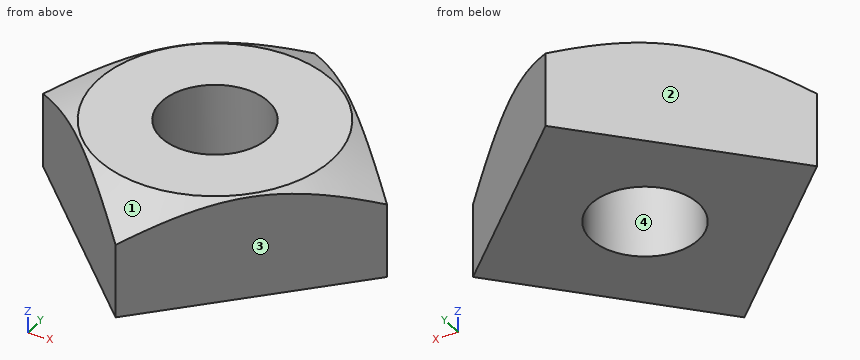
from build123d import *

# Parameters (mm, degrees)
SKETCH_7_R      = 1.229375
EXTRUDE_1_DEPTH = 2.4


with BuildPart() as part:
    # 草图7 → 凸台-拉伸1 (new body)
    with BuildSketch(Plane.XY):
        Polygon((-3.889087297, 0), (0, 3.889087297), (3.889087297, 0), (0, -3.889087297), align=None)
        Circle(SKETCH_7_R, mode=Mode.SUBTRACT)
    extrude(amount=-EXTRUDE_1_DEPTH)

    # 草图8 → 切除-旋转1 (revolve, cut)
    with BuildSketch(Plane(origin=(0, 0, 0), x_dir=(0, 0, -1), z_dir=(1, 0, 0))):
        Polygon((0.692820323, 3.889087297), (0, 2.689087297), (0, 3.889087297), align=None)
    revolve(axis=Axis((0, 0, 0), (0, 0, -1)), mode=Mode.SUBTRACT)


solid = part.part
For this review, take the finished solid that the model builds, in its own axes (mm). Face numbers are marked on the shaded views. Give positions to 0.01 mm unless a question says otherwise; leave off trailing zeros. Loops run counter-clockwise (first coordinate to the right, second up) from the corner with the lowest first, then second, coordinate; pieces in that order, holes last. Notation, with made-up numbers: (60.25, 55.25) -> (90.25, 55.25) arc R13 ccw to (90.25, 63.25) -> close; hole circle Ø7 at (78, 56.5). An arc over 180 degrees is marked (long way). One line per question, with ' | ' between items.
1) Insertion check: pin 1 Ø1 at (x, z) = (-1.5, -0.5) entering from -Y. The pin has a flat end and moves straight along its axis. Give the tip position at first contact, or say it passes through.
Resolved:
pin 1: stops at y = -2.89
2) To check wall thickness, follow probe 1 along Y at (x, z) = (0.5, -0.35); probe 2 along X at (y, z) = (-0.25, -0.6); probe 3 along Y at (x, z) = (0.5, -1.7). State the ranges of each line that lie inside material, in increasing order.
Resolved:
probe 1: y = -3.26 to -1.12, 1.12 to 3.26 | probe 2: x = -3.64 to -1.2, 1.2 to 3.64 | probe 3: y = -3.39 to -1.12, 1.12 to 3.39
3) We need section B-B (z = -0.6). Write out the cut boundary in (x, y), plus the area to 3 significant figures.
Resolved:
outline: (-3.72, -0.16) -> (-0.16, -3.72) arc R3.73 ccw to (0.16, -3.72) -> (3.72, -0.16) arc R3.73 ccw to (3.72, 0.16) -> (0.16, 3.72) arc R3.73 ccw to (-0.16, 3.72) -> (-3.72, 0.16) arc R3.73 ccw to start; hole circle Ø2.46 at (0, 0) | area: 25.4 mm2
4) We need section A-A (z = -1.8). Write out the cut boundary in (x, y).
Resolved:
outline: (-3.89, 0) -> (0, -3.89) -> (3.89, 0) -> (0, 3.89) -> close; hole circle Ø2.46 at (0, 0)
5) The part is to be moulded in two halves that separate along X. For the marked faces 1, 2, 3 and 4, say which applies: +X half, -X half, draft (parallel to the pull), parting line (faces both ways), or undercut.
Resolved:
face 1: parting line | face 2: -X half | face 3: +X half | face 4: undercut
